Read the model definition and answer for the solid it produces. Units are mm, in the model's axes. A direction names the side the tool comes from. Give positions to 0.01 mm unless a question says otherwise; leave off trailing zeros. Order: outer loops, then holes, each group sorted by start corner. A loop starts at its lowest first (then second) coordinate and runs counter-clockwise, first axis right, second up. Notation, with made-up numbers: (-38.75, -10) - (3.25, -10) arc R19 ccw to (3.25, 25) - close; hole circle Ø7 at (-8.75, 9). An arc over 180 degrees is marked (long way). Write each question's results on one line, items separated by ' | '. Start each with the question number.
Q1. Find section A-A on y = 5.5. Give the vertices of the cut face in (x, z).
Q2. For a pull along X with two mould halves and no side action, classify faces 1 (the face through (2.38, 8.07, -10.74)), 2 (the face through (7.493, 5.457, 0.33)), 3 (the face through (5, 8.828, -5)) as +X half, -X half, draft (parallel to the pull), parting line (faces both ways), or undercut.
Q3. A tool of negligible diameter and unlimited length cuts with its end or side. For faces 4 (the face through (6, 8, 0)), 5 (the face through (0, 3.978, 0)), 6 (the face through (-10.425, 4.89, 3.283)), from which of +Z, -Z, +X, -X, +Y, -Y can it reach the whole face along a straight path? Write none if from no direction.
Q4. Flat-ended cylindrical pins translate along their axes: P1, Ø2, axis at x = -7, z = -8, coming from the -Y side; P2, Ø12, axis at x = 7.5, z = -1, coming from the -Y side; P3, Ø4.5, axis at x = -2.5, z = 0.5, coming from the -Y side. Find the tip coordinate at first contact, or state that the pin passes through.
Q5. Find the intervals of material crossed by line 1 along Z through (x, y) = (0, 5.25); line 2 along Z through (x, y) = (0, 8.25); line 3 along Y through (x, z) = (9, -5.25), in increasing order. Write a range as from..to.
from build123d import *


with BuildPart() as part:
    # Sketch1 → Revolve1 (revolve)
    with BuildSketch(Plane.XY):
        Polygon((0, 0), (0, 8.828029189), (-11, 8.828029189), (-11, 7.328029189), (-10, 7.328029189), (-10, 5.828029189), (-10.929545371, 5.828029189), (-10.929545371, 3.978029189), align=None)
    revolve(axis=Axis((0, 0, 0), (0, 1, 0)))

    # Sketch2 → Cut-Revolve1 (revolve, cut)
    with BuildSketch(Plane.XY):
        Polygon((0, 3.978029189), (0, 9.978029189), (-6, 9.978029189), (-6, 6.978029189), (-7.5, 6.978029189), (-7.5, 3.978029189), align=None)
    revolve(axis=Axis((0, 3.978029189, 0), (0, 1, 0)), mode=Mode.SUBTRACT)


solid = part.part
Working result:
1) outline: circle Ø21.86 at (0, 0); hole circle Ø15 at (0, 0)
2) face 1: parting line | face 2: undercut | face 3: draft
3) face 4: +Y | face 5: none | face 6: -Y
4) P1: y = 3.51 | P2: y = 0.57 | P3: y = 0.11
5) line 1: -10.93..-7.5, 7.5..10.93 | line 2: -11..-6, 6..11 | line 3: 3.79..5.83, 7.33..8.83
